Design review of the part built by this model. Coordinates are the model's own, in mm. A direction names the side the tool comes from. Round coordinates to 2 decimals unless told otherwise and drop trailing zeros. Order: outer loops, then holes, each group sorted by start corner. A loop starts at its lowest first (then second) coordinate and runs counter-clockwise, first axis right, second up. Notation, with made-up numbers: M 53.25,83.25 L 80.25,83.25 A21 ccw 80.25,110.25 Z; hole C 8.5,-17.5 d8. An arc over 180 degrees is marked long. Use a Markdown table: item, result. Add a question column.
(1) The part is to be moulded in two halves that separate along X. For faces 4 (the face through (-20, 0, 0)), 5 (the face through (-1, 5, 17)), 6 (the face through (20, 0, 5)), 7 (the face through (15.6, 0, -12)), say which applies: released by +X, released by -X, zero draft, split by the parting line, or undercut.
(2) To check wall thickness, follow probe 1 along Y at (x, z) = (31.5, -19.3); probe 2 along Z at (x, y) = (0, 2.9); probe 3 along Z at (x, y) = (0, -3.45). State the ranges of each line that lie inside material, in increasing order. Write a range as from..to.
(3) Take a section at B-B (z = -13.5). Write out the cut boundary in (x, y).
(4) Take a section at D-D (z = -0.5). Write out the cut boundary in (x, y).
(5) For pin 1 (5 mm diameter, centred on x = -1, z = 28.5, fed in from +Y); pin 2 (11 mm diameter, centred on y = -1, z = 3.5, fed in from +X); pin 3 (9 mm diameter, centred on y = 32.5, z = -13, fed in from -X); pin 4 (6 mm diameter, centred on x = 30.5, y = 10, fed in from +Z), all flat-tipped, find the tip position at first contact; note any pin that passes through.
(6) Machinability: for faces 1 (the face through (21.25, 19, -14)), 2 (the face through (13.1, -0.1, 5.9)), 3 (the face through (-13, 0, 26)), which of the approach directions +Z, -Z, +X, -X, +Y, -Y give a long, thin tool a straight path to every point of the face, cutting with its end or side? Answer none if there is none.
(7) Take a section at A-A (y = 18). Write out the cut boundary in (x, z), then the cut area to 4 significant figures.
(8) Take a section at C-C (x = 0). Write out the cut boundary in (y, z).
Solid Edge part; units mm, degrees
sketch "Sketch1" plane through (0, 0, 0) normal (0, -1, 0) x (1, 0, 0)
  line L0 (-20, -20) -> (20, -20)
  line L1 (20, -20) -> (20, 20)
  line L2 (20, 20) -> (-20, 20)
  line L3 (-20, 20) -> (-20, -20)
extrude "Protrusion1" add sketch "Sketch1" along normal mid plane 10
sketch "Sketch2" plane through (0, -5, 0) normal (0, -1, 0) x (1, 0, 0)
  line L0 (-10.6, 3.4) -> (-15.6, 8.4)
  line L1 (-15.6, 15.6) -> (-15.6, 8.4)
  line L2 (15.6, 15.6) -> (-15.6, 15.6)
  line L3 (15.6, 8.4) -> (15.6, 15.6)
  line L4 (10.6, 3.4) -> (15.6, 8.4)
  line L5 (10.6, 3.4) -> (10.6, -3.4)
  line L6 (10.6, -3.4) -> (15.6, -8.4)
  line L7 (15.6, -15.6) -> (15.6, -8.4)
  line L8 (-15.6, -15.6) -> (15.6, -15.6)
  line L9 (-15.6, -8.4) -> (-15.6, -15.6)
  line L10 (-10.6, -3.4) -> (-15.6, -8.4)
  line L11 (-10.6, 3.4) -> (-10.6, -3.4)
  dimension "D1" = 10.6
extrude "Cutout1" cut sketch "Sketch2" against normal through all
sketch "Sketch3" plane through (0, -5, 0) normal (0, -1, 0) x (1, 0, 0)
  line L0 (-13, 32) -> (-13, 20)
  line L1 (-13, 20) -> (13, 20)
  line L2 (13, 20) -> (13, 32)
  arc A0 (13, 32) -> (-13, 32) centre (0, 32) ccw
extrude "ExtrudedProtrusion_2" add sketch "Sketch3" against normal blind 10
sketch "Sketch4" plane through (0, -5, 12.25) normal (0, -1, 0) x (1, 0, 0)
  circle A0 centre (0, 19.75) radius 11.2
extrude "ExtrudedCutout_2" cut sketch "Sketch4" against normal blind 5
sketch "Sketch5" plane through (0, 0, 32) normal (0, -1, 0) x (1, 0, 0)
  circle A0 centre (0, 0) radius 5.25
  circle A1 centre (0, 8) radius 1.6
  circle A2 centre (-8, 0) radius 1.6
  circle A3 centre (0, -8) radius 1.6
  circle A4 centre (8, 0) radius 1.6
extrude "Cutout2" cut sketch "Sketch5" against normal up to next
sketch "Sketch6" plane through (0, 5, 12.25) normal (0, 1, 0) x (-1, 0, 0)
  line L0 (-15.6, -27.85) -> (-15.6, -28.85)
  line L1 (-15.6, -28.85) -> (15.6, -28.85)
  line L2 (15.6, -28.85) -> (15.6, -27.85)
  line L3 (15.6, -27.85) -> (-15.6, -27.85)
extrude "ExtrudedCutout_12" cut sketch "Sketch6" against normal blind 209
sketch "Sketch7" plane through (0, 0, -20) normal (0, 0, -1) x (0, 1, 0)
  line L0 (-5, 20) -> (43, 20)
  line L1 (43, 20) -> (43, 43)
  line L2 (43, 43) -> (-5, 43)
  line L3 (-5, 43) -> (-5, 20)
extrude "ExtrudedProtrusion_7" add sketch "Sketch7" against normal blind 11
sketch "Sketch8" plane through (31.5, 19, -9) normal (0, 0, 1) x (-1, 0, 0)
  line L0 (-10.25, -22.75) -> (10.25, -22.75)
  line L1 (10.25, -22.75) -> (10.25, 22.75)
  line L2 (10.25, 22.75) -> (-10.25, 22.75)
  line L3 (-10.25, 22.75) -> (-10.25, -22.75)
extrude "ExtrudedCutout_17" cut sketch "Sketch8" against normal blind 9.9
sketch "Sketch9" plane through (31.5, 19, -18.9) normal (0, 0, 1) x (-1, 0, 0)
  circle A0 centre (0, 12.58) radius 8.1
  circle A1 centre (0, -12.63) radius 8.1
  line L0 (-10.25, 5) -> (-10.25, -5)
  line L1 (-10.25, -5) -> (-5.25, -5)
  line L2 (-5.25, -5) -> (-5.25, 5)
  line L3 (-5.25, 5) -> (-10.25, 5)
extrude "Cutout3" cut sketch "Sketch9" against normal up to next
Verdict:
| question | item | result |
|---|---|---|
| 1 | face 4 | released by -X |
| 1 | face 5 | zero draft |
| 1 | face 6 | released by +X |
| 1 | face 7 | undercut |
| 2 | probe 1 | y = -5..-1.68, 14.52..23.53, 39.73..43 |
| 2 | probe 2 | z = -20..-16.6, 15.6..22.4, 25.6..26.75, 37.25..38.4, 41.6..45 |
| 2 | probe 3 | z = -20..-16.6, 15.6..20.8, 43.2..45 |
| 3 | outline | M -20,-5 L -15.6,-5 L -15.6,5 L -20,5 Z; M 15.6,-5 L 43,-5 L 43,43 L 20,43 L 20,5 L 15.6,5 Z; hole M 21.25,-3.75 L 41.75,-3.75 L 41.75,41.75 L 21.25,41.75 Z |
| 4 | outline | M -20,-5 L -10.6,-5 L -10.6,5 L -20,5 Z; M 10.6,-5 L 20,-5 L 20,5 L 10.6,5 Z |
| 5 | pin 1 | stops at y = 5 |
| 5 | pin 2 | stops at x = 20 |
| 5 | pin 3 | stops at x = 20 |
| 5 | pin 4 | passes through |
| 6 | face 1 | +Z |
| 6 | face 2 | +Y, -Y |
| 6 | face 3 | +Z, -X, +Y, -Y |
| 7 | outline | M 20,-20 L 36.75,-20 L 36.75,-18.9 L 21.25,-18.9 L 21.25,-9 L 20,-9 Z; M 41.75,-20 L 43,-20 L 43,-9 L 41.75,-9 Z |
| 7 | area | 44.55 mm^2 |
| 8 | outline | M -5,-20 L 5,-20 L 5,-16.6 L -5,-16.6 Z; M -5,15.6 L 5,15.6 L 5,22.4 L 0,22.4 L 0,20.8 L -5,20.8 Z; M -5,43.2 L 0,43.2 L 0,41.6 L 5,41.6 L 5,45 L -5,45 Z; M 0,25.6 L 5,25.6 L 5,26.75 L 0,26.75 Z; M 0,37.25 L 5,37.25 L 5,38.4 L 0,38.4 Z |
